Read the model definition and answer for the solid it produces. Units are mm, in the model's axes. A direction names the side the tool comes from. Give positions to 0.01 mm unless a question says otherwise; leave off trailing zeros. Order: outer loops, then holes, each group sorted by start corner. A loop starts at its lowest first (then second) coordinate and runs counter-clockwise, first axis right, second up. Notation, with made-up numbers: (-32.75, 78) - (-8.75, 78) arc R9 ccw to (-8.75, 87) - close; hole circle Ø6 at (-18, 74). An arc over 180 degrees is marked (long way). Write item = value, one per line.
```python
from build123d import *

# Parameters (mm, degrees)
F0_W     = 100
F0_H     = 100
F1_DEPTH = 50
F2_R     = 15.625
F3_DEPTH = 37.5
F2_R_2   = 31.25
F4_DEPTH = 50


with BuildPart() as f1:
    # F0 (on Front) → F1 (new body, symmetric)
    with BuildSketch(Plane.XZ):
        Rectangle(F0_W, F0_H)
    extrude(amount=F1_DEPTH, both=True)

    # F2 (on face) → F3 (join, symmetric)
    with BuildSketch(Plane.XZ.offset(50)):
        Circle(F2_R)
    extrude(amount=F3_DEPTH, both=True)

    # F2 (on face) → F4 (join)
    with BuildSketch(Plane.XZ.offset(50)):
        Circle(F2_R_2)
        Circle(F2_R, mode=Mode.SUBTRACT)
    extrude(amount=-F4_DEPTH)


solid = f1.part
```
1. For faces 1 (the face through (-50, -1, -1)), 2 (the face through (-15.61, -69.01, 0.69)), determine the directions among +Z, -Z, +X, -X, +Y, -Y from which every point of the face is accessible in a straight line to the end or side of a thin tool.
Recorded:
face_1 = +Z, -Z, -X, +Y, -Y
face_2 = -Y
2. Section B-B (x = 0) is taken. Determine the outline of the cut face in (y, z) (3 decimals), and give its area (3 significant figures).
Recorded:
outline = (-87.5, -15.625) - (-50, -15.625) - (-50, -50) - (50, -50) - (50, 50) - (-50, 50) - (-50, 15.625) - (-87.5, 15.625) - close
area = 11,200 mm^2
3. Section C-C (y = -78) is taken. Determine the outline of the cut face in (x, z) (3 decimals), and give its area (3 significant figures).
Recorded:
outline = circle Ø31.25 at (0, 0)
area = 767 mm^2
4. A straight line is drawn through the part: L1, parallel to Y at x = -25, z = 30. Find the intervals that lie inside material, in ascending order. Write a range as [from, to].
Recorded:
L1 = [-50, 50]
5. Section A-A (z = 0) is taken. Determine the outline of the cut face in (x, y) (3 decimals), and give its area (3 significant figures).
Recorded:
outline = (-50, -50) - (-15.625, -50) - (-15.625, -87.5) - (15.625, -87.5) - (15.625, -50) - (50, -50) - (50, 50) - (-50, 50) - close
area = 11,200 mm^2
6. A flat-ended cylindrical pin translates along its axis: pin 1 (10 mm diameter, centred on y = -69, z = 10, fed in from -X). Find the tip coordinate at first contact, or state that the pin passes through.
Recorded:
pin_1 = -14.8
7. Section D-D (x = -32.5) is taken. Determine the outline of the cut face in (y, z).
Recorded:
outline = (-50, -50) - (50, -50) - (50, 50) - (-50, 50) - close
